```python
from build123d import *

# Parameters (mm, degrees)
F0_W     = 63.5
F0_H     = 19.05
F1_DEPTH = 6.35
F4_D     = 7.9375
F5_D     = 7.1374


with BuildPart() as f1:
    # F0 (on Front) → F1 (new body, symmetric)
    with BuildSketch(Plane.XZ):
        with Locations((0, 9.525)):
            Rectangle(F0_W, F0_H)
    extrude(amount=F1_DEPTH, both=True)

    # F4 (through all)
    with Locations(Plane.XZ.offset(6.35)):
        with Locations((0, 9.525)):
            Hole(F4_D / 2)

    # F5 (through all)
    with Locations(Plane.XY.offset(19.05)):
        with Locations((-22.225, 0), (22.225, 0)):
            Hole(F5_D / 2)


solid = f1.part
```
The listing builds one solid part. Answer for the finished solid, in the listing's coordinates (mm). Coordinates: 2 decimals unless noted, no trailing zeros. Write each loop counter-clockwise with the first axis right and the second up, starting at its lowest first coordinate (ties: lowest second). Pieces come first, ordered by that corner, then holes.
Q1. The mould has two halves that part along Z. Classify faces 1 (the flat face through (0, 0, 19.05)), 2 (the cylindrical face through (0.86, 0.09, 5.65)), 3 (the flat face through (-31.75, 0, 9)): released by +Z, released by -Z, zero draft, split by the parting line, or undercut.
Returned:
face 1: released by +Z
face 2: undercut
face 3: zero draft
Q2. Section A-A, the plane y = 0 is taken. Give the number of separate pieces and of enclosed holes in the cut face, then the cut area to 3 significant figures.
Returned:
separate pieces: 3
enclosed holes: 1
area: 888 mm2
Q3. Section C-C, the plane z = 16 is taken. Write down the section's boundary in (x, y) (3 decimals), then the cut area to 3 significant figures.
Returned:
outline: (-31.75, -6.35) - (31.75, -6.35) - (31.75, 6.35) - (-31.75, 6.35) - close; hole circle Ø7.137 at (-22.225, 0); hole circle Ø7.137 at (22.225, 0)
area: 726 mm2
Q4. Section B-B, the plane x = 0 is taken. Write down the section's boundary in (y, z), then the cut area to 3 significant figures.
Returned:
outline: (-6.35, 0) - (6.35, 0) - (6.35, 5.56) - (-6.35, 5.56) - close; (-6.35, 13.49) - (6.35, 13.49) - (6.35, 19.05) - (-6.35, 19.05) - close
area: 141 mm2
Q5. Find the intervals of material crossed by line 1 along Z through (x, y) = (0, 0.75); line 2 along X through (y, z) = (2.5, 4.75); line 3 along X through (y, z) = (1.5, 11.5), in increasing order.
Returned:
line 1: z = 0 to 5.56, 13.49 to 19.05
line 2: x = -31.75 to -24.77, -19.68 to 19.68, 24.77 to 31.75
line 3: x = -31.75 to -25.46, -18.99 to -3.44, 3.44 to 18.99, 25.46 to 31.75
